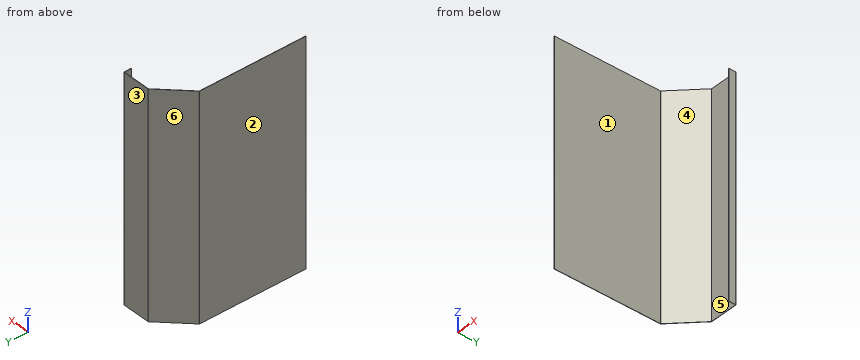
Autodesk Inventor part; units mm, degrees
ref_plane "YZ Plane" through (0, 0, 0) normal (1, 0, 0) x (0, 1, 0)
ref_plane "XZ Plane" through (0, 0, 0) normal (0, 1, 0) x (-1, 0, 0)
ref_plane "XY Plane" through (0, 0, 0) normal (0, 0, 1) x (1, 0, 0)
sketch "Sketch1" plane through (0, 0, 0) normal (0, 0, 1) x (1, 0, 0)
  line L0 (0, 650) -> (150, 800)
  line L1 (150, 800) -> (304, 800)
  line L2 (304, 800) -> (304, 760)
  line L3 (0, 650) -> (0, 70)
  point P0 (0, 0)
  dimension "d3" = 154
  dimension "d25" = 800
  dimension "d26" = 150
  dimension "d27" = 40
  dimension "d28" = 135
  dimension "d29" = 580
  dimension "d30" = 70
contour flange "Contour Flange1" sketch "Sketch1" thickness 1.6 bend radius 1.6 width 1200 along (0, 0, 1) mid plane no both sides no wall seen from (0, 360, 0) lies toward (1, 0, 0) curves L3 L0 L1 L2
bend "Bend1"
corner "Corner1"
equation "\"d4\" = Thickness"
equation "\"d5\" = BendReliefWidth"
equation "\"d6\" = BendReliefDepth"
equation "\"d7\" = MinimumRemnant"
equation "\"d8\" = TransitionRadius"
equation "\"d10\" = BendRadius"
equation "\"d12\" = CornerReliefSize"
equation "\"d13\" = GapSize"
equation "\"d14\" = JacobiRadiusSize"
equation "\"BendRadius\" = Thickness"
equation "\"BendReliefWidth\" = Thickness"
equation "\"BendReliefDepth\" = 0.5 * Thickness"
equation "\"CornerReliefSize\" = 4 * Thickness"
equation "\"MinimumRemnant\" = 2 * Thickness"
equation "\"TransitionRadius\" = BendRadius"
equation "\"JacobiRadiusSize\" = BendRadius"
equation "\"GapSize\" = Thickness"
properties part number "Front Cover with Cent point" material "Steel"
Input: part model. Units: mm. Frame: model coordinates. Face numbers are marked on the shaded views. A direction names the side the tool comes from. Coordinates: 2 decimals unless noted, no trailing zeros. Loops run counter-clockwise (first coordinate to the right, second up) from the corner with the lowest first, then second, coordinate; pieces in that order, holes last. Notation, with made-up numbers: (32.5, -17) - (86.5, -17) arc R19 ccw to (86.5, 4) - close; hole circle Ø10 at (-40, 61.5). An arc over 180 degrees is marked (long way). Answer in a Markdown table with one row per item. Add a question column.
Item 1: Section query B-B on x = 207. Return the cut outline in (y, z).
Item 2: Access query for the marked faces 1 and 2. Directions: +Z, -Z, +X, -X, +Y, -Y. A direction counts if a zero-diameter tool reaches every point of the face in a straight line with its end or side. Return the directions, or none.
Item 3: Mould query, pull axis X, two halves, no side actions, for the marked faces 3, 4, 5 and 6. Classes: released by +X, released by -X, zero draft, split by the parting line, or undercut.
Item 4: Contact query for flat-ended pins moving along their axis: P1, Ø2, axis at y = 324, z = 582, coming from the -X side; P2, Ø11, axis at y = 787, z = 428, coming from the -X side; P3, Ø8, axis at x = 132.5, z = 993.5, coming from the +Y side; P4, Ø1.5, axis at x = 78.5, z = 391, coming from the +Y side. Output: stop coordinate, or through.
Item 5: Line query: line 1 along X through (y, z) = (575.5, 610.5); line 2 along Y through (x, z) = (252, 1015); line 3 along Y through (x, z) = (134.5, 793). Output: solid intervals per line, ascending. Write a range as [from, to].
Item 6: Section query C-C on y = 616.5. Return the cut outline in (x, z), then the cut area to 3 significant figures.
Item 7: Section query A-A on z = 159.5. Return the cut outline in (x, y), then the cut area to 3 significant figures.
Recorded:
| question | item | result |
|---|---|---|
| 1 | outline | (798.4, 0) - (800, 0) - (800, 1200) - (798.4, 1200) - close |
| 2 | face 1 | +Z, -Z, +X, -Y |
| 2 | face 2 | +Z, -Z, -X, +Y, -Y |
| 3 | face 3 | zero draft |
| 3 | face 4 | undercut |
| 3 | face 5 | undercut |
| 3 | face 6 | released by -X |
| 4 | P1 | x = 0 |
| 4 | P2 | x = 131.5 |
| 4 | P3 | y = 786.5 |
| 4 | P4 | y = 729.25 |
| 5 | line 1 | [0, 1.6] |
| 5 | line 2 | [798.4, 800] |
| 5 | line 3 | [782.24, 784.5] |
| 6 | outline | (0, 0) - (1.6, 0) - (1.6, 1200) - (0, 1200) - close |
| 6 | area | 1,920 mm^2 |
| 7 | outline | (0, 70) - (1.6, 70) - (1.6, 648.67) arc R1.6 cw to (2.07, 649.81) - (150.19, 797.93) arc R1.6 cw to (151.33, 798.4) - (300.8, 798.4) arc R1.6 cw to (302.4, 796.8) - (302.4, 760) - (304, 760) - (304, 796.8) arc R3.2 ccw to (300.8, 800) - (151.33, 800) arc R3.2 ccw to (149.06, 799.06) - (0.94, 650.94) arc R3.2 ccw to (0, 648.67) - close |
| 7 | area | 1,570 mm^2 |
